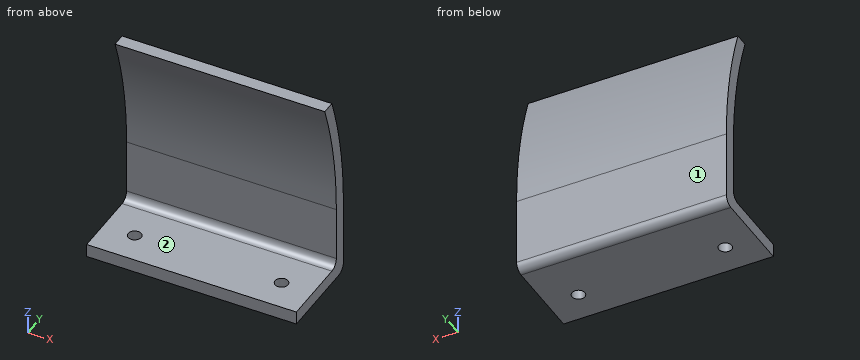
Autodesk Inventor part; units mm, degrees
ref_plane "YZ Plane" through (0, 0, 0) normal (1, 0, 0) x (0, 1, 0)
ref_plane "XZ Plane" through (0, 0, 0) normal (0, 1, 0) x (-1, 0, 0)
ref_plane "XY Plane" through (0, 0, 0) normal (0, 0, 1) x (1, 0, 0)
sketch "Sketch1" plane through (0, 0, 0) normal (1, 0, 0) x (0, 1, 0)
  line L0 (0, 0) -> (18, 0)
  line L1 (18, 0) -> (18, -3.175)
  line L2 (18, -3.175) -> (0, -3.175)
  line L3 (0, -3.175) -> (0, 0)
  line L4 (18, 0) -> (21.175, 0)
  line L5 (21.175, 0) -> (21.175, 15)
  line L6 (21.175, 15) -> (18, 15)
  line L7 (18, 15) -> (18, 0)
  line L8 (21.175, 0) -> (18, 0)
  line L9 (18, 0) -> (18, -3.175)
  line L10 (18, -3.175) -> (21.175, -3.175)
  line L11 (21.175, -3.175) -> (21.175, 0)
  arc A0 (21.175, 15) -> (15.9656, 44.5442) centre (-65.2066, 15) ccw
  line L12 (21.175, 15) -> (15.9656, 44.5442) construction
  line L13 (21.175, 15) -> (51.175, 15) construction
  line L14 (15.9656, 44.5442) -> (12.7906, 44.5442)
  arc A1 (18, 15) -> (12.7906, 44.5442) centre (-68.3816, 15) ccw
  line L15 (18, 15) -> (12.7906, 44.5442) construction
  line L16 (18, 15) -> (48, 15) construction
  dimension "d0" = 18
  dimension "d1" = 3.175
  dimension "d2" = 3.175
  dimension "d3" = 15
  dimension "d4" = 30
  dimension "d5" = 100
  dimension "d7" = 30
  dimension "d8" = 100
extrude "Extrusion1" add sketch "Sketch1" along normal mid plane 50
fillet "Fillet1" radius 2 2 edges at (0, 18, 0) (0, 21.175, -3.175)
sketch "Sketch2" plane through (25, 0, -3.175) normal (0, 0, -1) x (-1, 0, 0)
  line L0 (0, 0) -> (0, 19.175)
  line L1 (25, 0) -> (0, 0)
  line L2 (50, 19.175) -> (50, 0)
  line L3 (50, 7.5) -> (0, 7.5) construction
  circle A0 centre (7.5, 7.5) radius 1.55
  circle A1 centre (42.5, 7.5) radius 1.55
  dimension "d12" = 7.5
  dimension "d13" = 3.1
  dimension "d14" = 3.1
  dimension "d15" = 7.5
  dimension "d16" = 7.5
extrude "Extrusion2" cut sketch "Sketch2" against normal blind 10
properties part number "PolyWedge" material "PC/ABS Plastic"
Could you check a few things on this model? Use its own coordinates, in mm. Face numbers are marked on the shaded views. A direction names the side the tool comes from. Give positions to 0.01 mm unless a question says otherwise; leave off trailing zeros. Order: outer loops, then holes, each group sorted by start corner. A loop starts at its lowest first (then second) coordinate and runs counter-clockwise, first axis right, second up.
Q1. If I drill on line 1 along Y through (x, z) = (17.5, -1.05) (3 decimals); line 2 along Z through (x, y) = (15, 9.5) (3 decimals); line 3 along Y through (x, z) = (-2, 11) (3 decimals), over which ranges is the centre line in solid material (lowest first)?
Q2. Suppose I cut it at D-D, the plane z = 23.5. Write out the boundary of the cut face in (x, y), and give its area (3 significant figures).
Q3. For the marked faces 1 and 2, which set-ups out of +Z, -Z, +X, -X, +Y, -Y let a thin tool reach every point of the face, with its end or its side?
Q4. Suppose I cut it at A-A, the plane x = 17.5. Write out the boundary of the cut face in (y, z) (3 decimals), and give its area (3 significant figures).
Q5. Suppose I cut it at B-B, the plane x = 12.5. Write out the boundary of the cut face in (y, z) (3 decimals), and give its area (3 significant figures).
Q6. I'm going to push flat-ended pins straight in: P1, Ø1, axis at x = -17.5, y = 3, coming from the +Z side; P2, Ø4, axis at x = 11, z = 6.5, coming from the -Y side. Where does each tip first touch, or does it pass through?
Q7. Suppose I cut it at C-C, the plane y = 2. Write out the boundary of the cut face in (x, z) (3 decimals), and give its area (3 significant figures).
Solution:
1. line 1: y = 0 to 5.95, 9.05 to 21.175
1. line 2: z = -3.175 to 0
1. line 3: y = 18 to 21.175
2. outline: (-25, 17.58) - (25, 17.58) - (25, 20.76) - (-25, 20.76) - close
2. area: 159 mm2
3. face 1: +Z, -Z, +X, -X, +Y
3. face 2: +X, -X, -Y
4. outline: (0, -3.175) - (5.95, -3.175) - (5.95, 0) - (0, 0) - close; (9.05, -3.175) - (19.175, -3.175) arc R2 ccw to (21.175, -1.175) - (21.175, 15) arc R86.383 ccw to (15.966, 44.544) - (12.791, 44.544) arc R86.383 cw to (18, 15) - (18, 2) arc R2 cw to (16, 0) - (9.05, 0) - close
4. area: 199 mm2
5. outline: (0, -3.175) - (19.175, -3.175) arc R2 ccw to (21.175, -1.175) - (21.175, 15) arc R86.383 ccw to (15.966, 44.544) - (12.791, 44.544) arc R86.383 cw to (18, 15) - (18, 2) arc R2 cw to (16, 0) - (0, 0) - close
5. area: 209 mm2
6. P1: stops at z = 0
6. P2: stops at y = 18
7. outline: (-25, -3.175) - (25, -3.175) - (25, 0) - (-25, 0) - close
7. area: 159 mm2
